from build123d import *

# Parameters (mm, degrees)
BOSS_EXTRUDE1_DEPTH      = 100
SHELL1_T                 = -1
SKETCH2_W                = 28
SKETCH2_H                = 18
CUT_EXTRUDE1_DEPTH       = 1
FILLET1_R                = 5
M3_CLEARANCE_HOLE1_D     = 3.6
M3_CLEARANCE_HOLE1_DEPTH = 10
M3_CLEARANCE_HOLE1_TIP   = 1.081549114


with BuildPart() as part:
    # Sketch1 → Boss-Extrude1 (new, symmetric)
    with BuildSketch(Plane.XY):
        Polygon((0, 0), (515, 0), (515, 30), (440, 75), (0, 75), align=None)
    extrude(amount=BOSS_EXTRUDE1_DEPTH, both=True)

    # Shell1
    shell1_openings = [part.faces().sort_by_distance(p)[0] for p in [
        (257.5, 0, 0),
    ]]
    offset(amount=SHELL1_T, openings=shell1_openings, kind=Kind.INTERSECTION)

    # Sketch2 → Cut-Extrude1 (cut)
    with BuildSketch(Plane.XY.offset(100)):
        with Locations((30, 45)):
            Rectangle(SKETCH2_W, SKETCH2_H)
    extrude(amount=-CUT_EXTRUDE1_DEPTH, mode=Mode.SUBTRACT)

    # Fillet1
    fillet1_edges = [part.edges().sort_by_distance(p)[0] for p in [
        (16, 36, 99.5),
        (16, 54, 99.5),
        (44, 54, 99.5),
        (44, 36, 99.5),
    ]]
    fillet(fillet1_edges, radius=FILLET1_R)

    # M3 Clearance Hole1
    with Locations(Plane.XY.offset(100)):
        with Locations((10, 45.046525162), (50, 45.046525162)):
            Hole(M3_CLEARANCE_HOLE1_D / 2, depth=M3_CLEARANCE_HOLE1_DEPTH)
            with Locations((0, 0, -(M3_CLEARANCE_HOLE1_DEPTH + M3_CLEARANCE_HOLE1_TIP / 2))):  # 118° drill point
                Cone(0, M3_CLEARANCE_HOLE1_D / 2, M3_CLEARANCE_HOLE1_TIP, mode=Mode.SUBTRACT)


solid = part.part
Work out the finished part from the listing and answer in its coordinate system (mm). A direction names the side the tool comes from. Give positions to 0.01 mm unless a question says otherwise; leave off trailing zeros. Loops run counter-clockwise (first coordinate to the right, second up) from the corner with the lowest first, then second, coordinate; pieces in that order, holes last. Notation, with made-up numbers: (-15, 22) - (-5, 22) arc R5 cw to (-5, 26) - close; hole circle Ø2 at (13.25, 56). An arc over 180 degrees is marked (long way). Answer in a Markdown table with one row per item. Add a question column.
Q1. The part is cut by section B-B (z = -26). Determine the outline of the cut face in (x, y).
Q2. Each of these flat-tipped pins is pushed along its axis until it touches: P1, Ø2, axis at y = 38, z = -48, coming from the +X side; P2, Ø1, axis at x = 443, z = -12.5, coming from the -Y side; P3, Ø0.8, axis at y = 47, z = 99.5, coming from the +X side. Where does it stop, or does it pass through?
Q3. The part is cut by section D-D (y = 69.5). Determine the outline of the cut face in (x, z), and give its area (3 significant figures).
Q4. A tool of negligible diameter and unlimited length cuts with its end or side. For faces 1 (the flat face through (223, 74, 1)), 2 (the flat face through (254, 38, -100)), from which of +Z, -Z, +X, -X, +Y, -Y can it reach the whole face along a straight path? Write none if from no direction.
Q5. Consider line 1 along X through (y, z) = (19.5, 80.5); line 2 along Z through (x, y) = (60, 6); line 3 along Y through (x, z) = (50, 99.5). Determine where each line is inside the solid, lowest interval first.
Q6. The part is cut by section A-A (y = 16.5). Determine the outline of the cut face in (x, z).
Q7. The part is cut by section C-C (x = 330). Determine the outline of the cut face in (y, z).
Solution:
| question | item | result |
|---|---|---|
| 1 | outline | (0, 0) - (1, 0) - (1, 74) - (439.72, 74) - (514, 29.43) - (514, 0) - (515, 0) - (515, 30) - (440, 75) - (0, 75) - close |
| 2 | P1 | stops at x = 503.33 |
| 2 | P2 | stops at y = 71.73 |
| 2 | P3 | stops at x = 487.33 |
| 3 | outline | (0, -100) - (449.17, -100) - (449.17, 100) - (0, 100) - close; hole (1, -99) - (447.22, -99) - (447.22, 99) - (1, 99) - close |
| 3 | area | 1,480 mm² |
| 4 | face 1 | -Y |
| 4 | face 2 | -Z, +X, -X, +Y, -Y |
| 5 | line 1 | x = 0 to 1, 514 to 515 |
| 5 | line 2 | z = -100 to -99, 99 to 100 |
| 5 | line 3 | y = 0 to 43.25, 46.85 to 75 |
| 6 | outline | (0, -100) - (515, -100) - (515, 100) - (0, 100) - close; hole (1, -99) - (514, -99) - (514, 99) - (1, 99) - close |
| 7 | outline | (0, -100) - (75, -100) - (75, 100) - (0, 100) - (0, 99) - (74, 99) - (74, -99) - (0, -99) - close |
